CAD build for the part. Positions are in the model's coordinates, mm. A direction names the side the tool comes from. Coordinates: 2 decimals unless noted, no trailing zeros. Order: outer loops, then holes, each group sorted by start corner. A loop starts at its lowest first (then second) coordinate and runs counter-clockwise, first axis right, second up. Notation, with made-up numbers: (-22.75, -36.75) - (-11.75, -36.75) arc R13 cw to (-11.75, -20.75) - close; hole circle Ø10 at (-26.75, -27). An arc over 180 degrees is marked (long way). Return JSON: item names as keys, results as strings.
from build123d import *

# Parameters (mm, degrees)
SKETCH_5_R          = 15
EXTRUDE_5_DEPTH     = 25
SKETCH_6_R          = 10
SKETCH_6_R_2        = 15
EXTRUDE_6_DEPTH     = 8
SKETCH_8_R          = 7.5
EXTRUDE_7_DEPTH     = 5
SKETCH_16_R         = 15
CUT_EXTRUDE_1_DEPTH = 10
EXTRUDE_14_DEPTH    = 5


with BuildPart() as part:
    # 스케치5 → 보스-돌출5 (new body)
    with BuildSketch(Plane.XY):
        Circle(SKETCH_5_R)
    extrude(amount=-EXTRUDE_5_DEPTH)

    # 스케치6 → 보스-돌출6 (add)
    with BuildSketch(Plane(origin=(0, 0, -25), x_dir=(-1, 0, 0), z_dir=(0, 0, -1))):
        with BuildLine():
            ThreePointArc((-15, 0), (0, -15), (15, 0))
            Line((15, 0), (-15, 0))
        make_face()
        with BuildLine():
            Line((-15, 0), (15, 0))
            ThreePointArc((15, 0), (0, 15), (-15, 0))
        make_face()
        with BuildLine():
            ThreePointArc((-15, 0), (0, 15), (15, 0))
            Line((15, 0), (15, 30))
            Line((15, 30), (10, 30))
            ThreePointArc((10, 30), (0, 20), (-10, 30))
            Line((-10, 30), (-15, 30))
            Line((-15, 30), (-15, 0))
        make_face()
        with Locations((0, 30)):
            Circle(SKETCH_6_R)
        with BuildLine():
            Line((15, 30), (-15, 30))
            ThreePointArc((-15, 30), (0, 45), (15, 30))
        make_face()
        with Locations(Location((0, 0, 0), (0, 0, 180))):
            Circle(SKETCH_6_R_2)
    extrude(amount=EXTRUDE_6_DEPTH)

    # 스케치8 → 보스-돌출7 (add)
    with BuildSketch(Plane(origin=(0, 0, -33), x_dir=(-1, 0, 0), z_dir=(0, 0, -1))):
        with Locations((0, 30)):
            Circle(SKETCH_8_R)
    extrude(amount=EXTRUDE_7_DEPTH)

    # 스케치16 → 컷-돌출1 (cut)
    with BuildSketch(Plane.XY):
        Circle(SKETCH_16_R)
        Polygon((0, 6.180339887), (-5.877852523, 1.909830056), (-3.63271264, -5), (3.63271264, -5), (5.877852523, 1.909830056), align=None, mode=Mode.SUBTRACT)
    extrude(amount=-CUT_EXTRUDE_1_DEPTH, mode=Mode.SUBTRACT)

    # 스케치19 → 보스-돌출14 (add)
    with BuildSketch(Plane(origin=(0, 0, -38), x_dir=(-1, 0, 0), z_dir=(0, 0, -1))):
        Polygon((0, 34.94427191), (-4.702282018, 31.527864045), (-2.906170112, 26), (2.906170112, 26), (4.702282018, 31.527864045), align=None)
    extrude(amount=EXTRUDE_14_DEPTH)


solid = part.part
Item 1: Which spindle directions (+Z, -Z, +X, -X, +Y, -Y) get a long thin tool onto all of the face, cutting with end or side? Do faces 1 (the flat face through (3.817, 28.803, -40.465)), 2 (the flat face through (-2.4, 33.2, -40.5)), 3 (the flat face through (3, 4, -5)), 4 (the cylindrical face through (1.63, 22.68, -35.47)). Say none if no direction does.
Findings below:
{"face 1": "-Z, +X, -Y", "face 2": "-Z, -X, +Y", "face 3": "+Z, +X, +Y", "face 4": "-Z"}
Item 2: Wall check: L1, parallel to Z at x = 14, y = 24; L2, parallel to Z at x = -11, y = -1; L3, parallel to Y at x = 0, z = -12.5. Give the ranges that are in metal, low to high. Write a range as [from, to].
Findings below:
{"L1": "z = [-33, -25]", "L2": "z = [-33, -10]", "L3": "y = [-15, 15]"}
Item 3: Band-saw the part on B-B, the plane x = 11. List the corners of the cut face in (y, z), then the cut area to 3 significant figures.
Findings below:
{"outline": "(-10.2, -33) - (40.2, -33) - (40.2, -25) - (10.2, -25) - (10.2, -10) - (-10.2, -10) - close", "area": "709 mm²"}
Item 4: Band-saw the part on C-C, the plane z = -24. List the corners of the cut face in (x, y), then the cut area to 3 significant figures.
Findings below:
{"outline": "circle Ø30 at (0, 0)", "area": "707 mm²"}
Item 5: Band-saw the part on D-D, the plane y = -6. List the corners of the cut face in (x, z).
Findings below:
{"outline": "(-13.75, -33) - (13.75, -33) - (13.75, -10) - (-13.75, -10) - close"}
Item 6: Drop flat-ended pins along their axis: P1, Ø2.5, axis at x = -1, z = -41, coming from the -Y side; P2, Ø6, axis at y = 12, z = -12.5, coming from the -X side; P3, Ø2, axis at x = 5, y = 15.5, coming from the -Z side. Give the stop position or say it passes through.
Findings below:
{"P1": "stops at y = 26", "P2": "stops at x = -12", "P3": "stops at z = -33"}
Item 7: Band-saw the part on A-A, the plane z = -29. List the corners of the cut face in (x, y).
Findings below:
{"outline": "(-15, 0) arc R15 ccw to (15, 0) - (15, 30) arc R15 ccw to (-15, 30) - close"}
